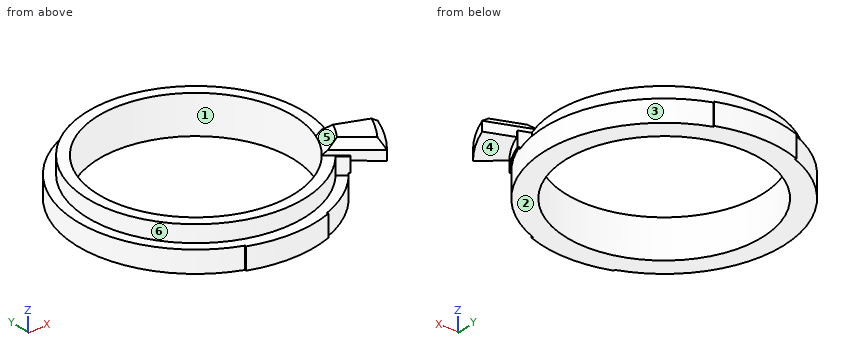
Autodesk Inventor part; units mm, degrees
ref_plane "YZ Plane" through (0, 0, 0) normal (1, 0, 0) x (0, 1, 0)
ref_plane "XZ Plane" through (0, 0, 0) normal (0, 1, 0) x (-1, 0, 0)
ref_plane "XY Plane" through (0, 0, 0) normal (0, 0, 1) x (1, 0, 0)
sketch "スケッチ1" plane through (0, 0, 0) normal (0, 0, 1) x (1, 0, 0)
  circle A0 centre (0, 0) radius 24.9
  circle A1 centre (0, 0) radius 20.25
  dimension "d0" = 4.65
  dimension "d1" = 40.5
extrude "押し出し1" add sketch "スケッチ1" along normal blind 8
sketch "スケッチ2" plane through (0, 0, 0) normal (0, 0, 1) x (1, 0, 0)
  circle A0 centre (0, 0) radius 24.9
  arc A1 (8.4137, -23.1164) -> (8.4137, 23.1164) centre (0, 0) ccw
  line L0 (0, -35.35) -> (0, 35.35)
  line L1 (8.4137, 23.1164) -> (8.5163, 23.3983)
  line L2 (8.4137, -23.1164) -> (8.5163, -23.3983)
  line L3 (-35.35, 0) -> (35.35, 0)
  point P0 (24.6, 0)
  dimension "d4" = 0.3
  dimension "d5" = 140
extrude "押し出し2" cut sketch "スケッチ2" along normal blind 5 contours L3 A1 L1 A0 | A0 L2 A1 L3
mirror "ミラー1" about plane through (0, 0, 0) normal (1, 0, 0) of "押し出し2"
sketch "スケッチ4" plane through (0, 0, 8) normal (0, 0, 1) x (1, 0, 0)
  circle A0 centre (0, 0) radius 24.9
  line L0 (21.7123, -12.5356) -> (0, 0)
  line L1 (-36.1071, 0) -> (39.8926, 0)
  arc A1 (23.8972, -19.3516) -> (28.7076, -11.0198) centre (0, 0) ccw
  arc A2 (17.6801, -14.317) -> (21.239, -8.1529) centre (0, 0) ccw
  line L2 (23.8972, -19.3516) -> (17.6801, -14.317)
  line L3 (21.239, -8.1529) -> (28.7076, -11.0198)
  circle A3 centre (0, 0) radius 20.25
  point P0 (26.6303, -15.375)
  point P1 (19.7021, -11.375)
  dimension "d18" = 30
  dimension "d46" = 2.5
  dimension "d47" = 8
  dimension "d48" = 18
extrude "押し出し7" add sketch "スケッチ4" along normal blind 2.5 and the other way blind 1 contours L3 A1 L2 A0 | A0 L0 A2 L3 | L2 A2 L0 A0
chamfer "面取り4" distance 2.5 angle 45 1 edges at (19.7021, -11.375, 8)
sketch "スケッチ7" plane through (0, 0, 8) normal (0, 0, 1) x (1, 0, 0)
  arc A0 (23.3983, -8.5163) -> (19.0745, -16.0054) centre (0, 0) ccw
  arc A1 (21.1431, -7.6955) -> (17.236, -14.4627) centre (0, 0) ccw
  arc A2 (18.905, -7.257) -> (15.7372, -12.7437) centre (0, 0) ccw
  line L0 (21.1431, -7.6955) -> (23.3983, -8.5163)
  arc A3 (23.2462, -8.9234) -> (19.3509, -15.6701) centre (0, 0) ccw
  line L1 (17.236, -14.4627) -> (19.0745, -16.0054)
  line L2 (17.6801, -14.317) -> (23.8972, -19.3516)
  line L3 (28.7076, -11.0198) -> (21.239, -8.1529)
  dimension "d57" = 1
  dimension "d59" = 2.4
  dimension "d65" = 1
extrude "押し出し8" cut sketch "スケッチ7" against normal blind 3.5
chamfer "面取り5" distance 1.5 angle 45 3 edges at (26.6303, -15.375, 10.5) (24.9733, -9.5863, 10.5) (20.7887, -16.8343, 10.5)
properties part number "ring"
The model under review builds one solid part; all positions refer to its coordinate system, in mm. Face numbers are marked on the shaded views. A direction names the side the tool comes from. Coordinates: 2 decimals unless noted, no trailing zeros. Write each loop counter-clockwise with the first axis right and the second up, starting at its lowest first coordinate (ties: lowest second). Pieces come first, ordered by that corner, then holes.
1) We need section C-C on x = -21. State the section outline as (y, z) points, then the cut area to 3 significant figures.
2) We need section A-A on x = 0. State the section outline as (y, z) points, then the cut area to 3 significant figures.
3) To check wall thickness, follow probe 1 along Y at (x, z) = (0, 3.5); probe 2 along Y at (x, z) = (0, 6.25); probe 3 along X at (y, z) = (2.5, 1). State the ranges of each line that lie inside material, in increasing order.
4) Machinability: for the marked faces 4, 5 and 6, which of the approach directions +Z, -Z, +X, -X, +Y, -Y give a long, thin tool a straight path to every point of the face, cutting with its end or side? Answer none if there is none.
5) Clearance check with flat-ended pins moving along their axes: pin 1 Ø3 at (x, y) = (24.5, -13.5) entering from -Z; pin 2 Ø1.5 at (y, z) = (-13, 5) entering from -X; pin 3 Ø5 at (x, y) = (3, 18.5) entering from +Z. State where each tip first meets the part, or that it passes through.
6) The part is to be moulded in two halves that separate along X. For the marked faces 1, 2 and 3, say which applies: pulls with the +X half, pulls with the -X half, needs draft (parallel to the pull), parting line crosses it, or undercut.
7) We need section B-B on y = 0. State the section outline as (x, z) points.
Answer list:
1. outline: (-12.81, 0) - (12.81, 0) - (12.81, 4.5) - (8.08, 4.5) - (8.08, 8) - (-8.08, 8) - (-8.08, 4.5) - (-12.81, 4.5) - close
1. area: 172 mm2
2. outline: (-24.9, 0) - (-20.25, 0) - (-20.25, 8) - (-22.5, 8) - (-22.5, 4.5) - (-24.9, 4.5) - close; (20.25, 0) - (24.9, 0) - (24.9, 4.5) - (22.5, 4.5) - (22.5, 8) - (20.25, 8) - close
2. area: 57.6 mm2
3. probe 1: y = -24.9 to -20.25, 20.25 to 24.9
3. probe 2: y = -22.5 to -20.25, 20.25 to 22.5
3. probe 3: x = -24.47 to -20.1, 20.1 to 24.47
4. face 4: -Z, +X, -Y
4. face 5: +Z, -X, +Y
4. face 6: +Z
5. pin 1: stops at z = 7
5. pin 2: stops at x = -21.22
5. pin 3: stops at z = 8
6. face 1: undercut
6. face 2: needs draft
6. face 3: pulls with the +X half
7. outline: (-24.6, 0) - (-20.25, 0) - (-20.25, 8) - (-22.5, 8) - (-22.5, 4.5) - (-24.6, 4.5) - close; (20.25, 0) - (24.6, 0) - (24.6, 4.5) - (22.5, 4.5) - (22.5, 8) - (20.25, 8) - close
